Check sheet for the modelled part. Datum: model origin and axes. Units: mm. A direction names the side the tool comes from. Coordinates: 2 decimals unless noted, no trailing zeros. Loops run counter-clockwise (first coordinate to the right, second up) from the corner with the lowest first, then second, coordinate; pieces in that order, holes last. Notation, with made-up numbers: (-4, 68.25) -> (27, 68.25) arc R17 cw to (27, 99.25) -> close; hole circle Ø1 at (34, 49.25). An arc over 180 degrees is marked (long way). Use one line per item in the form item = value.
Autodesk Inventor part; units mm, degrees
ref_plane "Start plane" through (0, 0, -10) normal (0, 0, 1) x (1, 0, 0)
ref_plane "End plane" through (0, 0, 110) normal (0, 0, 1) x (1, 0, 0)
ref_plane "Work Plane11" through (-6, 4, -10) normal (0.7071, 0, -0.7071) x (-0.7071, 0, -0.7071)
ref_plane "Start plane" through (0, 0, -10) normal (0, 0, 1) x (1, 0, 0)
ref_plane "End plane" through (0, 0, 110) normal (0, 0, 1) x (1, 0, 0)
sketch "Sketch" plane through (0, 0, 0) normal (0, 0, 1) x (1, 0, 0)
  line L0 (-3, 0.5) -> (-3, 12)
  line L1 (-6, 14) -> (-5, 14)
  line L2 (-6, -6) -> (-6, 14)
  line L3 (-6, -6) -> (14, -6)
  line L4 (14, -5) -> (14, -6)
  line L5 (0.5, -3) -> (12, -3)
  arc A0 (-3, 0.5) -> (0.5, -3) centre (0.5, 0.5) ccw
  arc A1 (-3, 12) -> (-5, 14) centre (-5, 12) ccw
  arc A2 (14, -5) -> (12, -3) centre (12, -5) ccw
  line L6 (0, 18.4971) -> (0, -10.0828) construction
  line L7 (-10.0828, 0) -> (18.4971, 0) construction
  point P0 (-3, -3)
  point P1 (-3, 14)
  point P2 (14, -3)
  dimension "d4" = 20
  dimension "d6" = 20
  dimension "d8" = 3
  dimension "d10" = 3
  dimension "d17" = 3.5
  dimension "d18" = 2
  dimension "d19" = 6
  dimension "d20" = 6
extrude "Body" add sketch "Sketch" along normal up to surface (120 mm away) from surface at -10
sketch "Sketch3" plane through (0, 0, 0) normal (0, 0, 1) x (1, 0, 0)
  line L0 (0, 0) -> (10, 0)
ref_plane "Work Plane10" through (0, 0, 0) normal (0, -1, 0) x (1, 0, 0)
sketch "Sketch4" plane through (0, 0, 0) normal (0, -1, 0) x (1, 0, 0)
  line L0 (-2, -10) -> (12, -10)
  line L1 (-2, 110) -> (12, 110)
  dimension "d24" = 120
ref_plane "Work Plane11" through (-6, 4, -10) normal (0.7071, 0, -0.7071) x (-0.7071, 0, -0.7071)
split "Split1" plane through (-6, 4, -10) removes the side toward (0.7071, 0, -0.7071)
ref_plane "Work Plane12" through (-6, 4, 110) normal (0.7071, 0, 0.7071) x (0.7071, 0, -0.7071)
split "Split2" plane through (-6, 4, 110) removes the side toward (0.7071, 0, 0.7071)
equation "\"d4\" = b"
equation "\"d6\" = b"
equation "\"d17\" = R"
equation "\"d18\" = R1"
equation "\"d19\" = ex"
equation "\"d20\" = d19"
equation "\"d11\" = G_L"
equation "\"b\" = 20"
equation "\"ParT\" = 3"
equation "\"R\" = 3.5"
equation "\"R1\" = 2"
equation "\"G_L\" = d24"
equation "\"ex\" = 6"
equation "\"G_OFFSET_START\" = 10"
equation "\"G_OFFSET_END\" = 10"
equation "\"d21\" = -G_OFFSET_START"
equation "\"d22\" = G_OFFSET_END + B_L"
equation "\"B_L\" = 100"
properties part number "ISO 657-1 - L20x20x3-120" material "Stainless Steel"
(1) Section check B-B, the plane x = 4.25. Record the boundary of the cut face in (y, z), plus the area to 4 significant figures.
Established:
outline = (-6, 0.25) -> (-3, 0.25) -> (-3, 99.75) -> (-6, 99.75) -> close
area = 298.5 mm²
(2) Go/stop test with flat-tipped pins: P1, Ø6, axis at y = 10.5, z = 54.5, coming from the +X side; P2, Ø4, axis at y = -0.5, z = 87, coming from the +X side; P3, Ø5, axis at x = 3, y = 0, coming from the -Z side; P4, Ø2, axis at x = 7, z = 53.5, coming from the +Y side. Record where each tip stops, or that it passes through.
Established:
P1 = -3
P2 = -1.3
P3 = through
P4 = -3
(3) Section check C-C, the plane z = 4.5. Record the boundary of the cut face in (x, y).
Established:
outline = (-6, -6) -> (8.5, -6) -> (8.5, -3) -> (0.5, -3) arc R3.5 cw to (-3, 0.5) -> (-3, 12) arc R2 ccw to (-5, 14) -> (-6, 14) -> close
(4) Section check D-D, the plane y = 6. Record the boundary of the cut face in (x, z).
Established:
outline = (-6, -10) -> (-3, -7) -> (-3, 107) -> (-6, 110) -> close
(5) Tool access check on faces 1 (the flat face through (-0.5, -3.5, 104.5)), 2 (the flat face through (-3, 6, 49)). Record the directions out of +Z, -Z, +X, -X, +Y, -Y that give a thin tool (end or side, any length) a straight path to the whole face; none if there is none.
Established:
face_1 = +Z, +X, +Y, -Y
face_2 = +Z, -Z, +X, +Y
(6) Section check A-A, the plane z = 67.5. Record the boundary of the cut face in (x, y), plus the area to 3 significant figures.
Established:
outline = (-6, -6) -> (14, -6) -> (14, -5) arc R2 ccw to (12, -3) -> (0.5, -3) arc R3.5 cw to (-3, 0.5) -> (-3, 12) arc R2 ccw to (-5, 14) -> (-6, 14) -> close
area = 112 mm²
(7) Scan lines: line 1 along Y through (x, z) = (11.75, 34); line 2 along Y through (x, z) = (-0.25, 71). Record each from-to range of solid material in increasing order.
Established:
line_1 = -6 to -3
line_2 = -6 to -2.92
